```python
from build123d import *

# Parameters (mm, degrees)
SKETCH1_R           = 3.66
BOSS_EXTRUDE1_DEPTH = 1.25
SKETCH2_R           = 2.4
BOSS_EXTRUDE2_DEPTH = 0.8
SKETCH3_R           = 2.25
BOSS_EXTRUDE3_DEPTH = 6.3
BOSS_EXTRUDE4_DEPTH = 2.95
SKETCH5_R           = 0.775
CUT_EXTRUDE4_DEPTH  = 0.2
CUT_EXTRUDE7_DEPTH  = 10.77


with BuildPart() as part:
    # Sketch1 → Boss-Extrude1 (new body)
    with BuildSketch(Plane(origin=(0, 0, 0), x_dir=(1, 0, 0), z_dir=(0, 1, 0))):
        with Locations(Location((0, 0, 0), (0, 0, 270))):
            Circle(SKETCH1_R)
    extrude(amount=BOSS_EXTRUDE1_DEPTH)

    # Sketch2 → Boss-Extrude2 (add)
    with BuildSketch(Plane(origin=(0, 1.25, 0), x_dir=(1, 0, 0), z_dir=(0, 1, 0))):
        with Locations(Location((0, 0, 0), (0, 0, 270))):
            Circle(SKETCH2_R)
    extrude(amount=BOSS_EXTRUDE2_DEPTH)

    # Sketch3 → Boss-Extrude3 (add)
    with BuildSketch(Plane(origin=(0, 2.05, 0), x_dir=(1, 0, 0), z_dir=(0, 1, 0))):
        with Locations(Location((0, 0, 0), (0, 0, 270))):
            Circle(SKETCH3_R)
    extrude(amount=BOSS_EXTRUDE3_DEPTH)

    # Sketch4 → Boss-Extrude4 (add)
    with BuildSketch(Plane(origin=(0, 8.35, 0), x_dir=(1, 0, 0), z_dir=(0, 1, 0))):
        Polygon((-2.222798536, 0), (-1.111399268, -1.925), (1.111399268, -1.925), (2.222798536, 0), (1.111399268, 1.925), (-1.111399268, 1.925), align=None)
    extrude(amount=BOSS_EXTRUDE4_DEPTH)

    # Sketch5 → Cut-Extrude4 (cut)
    with BuildSketch(Plane(origin=(0, 11.3, 0), x_dir=(1, 0, 0), z_dir=(0, 1, 0))):
        with Locations(Location((0, 0, 0), (0, 0, 270))):
            Circle(SKETCH5_R)
    extrude(amount=-CUT_EXTRUDE4_DEPTH, mode=Mode.SUBTRACT)

    # Sketch7 → Cut-Extrude7 (cut)
    with BuildSketch(Plane.XZ):
        Polygon((-0.95, 0), (-0.475, -0.822724134), (0.475, -0.822724134), (0.95, 0), (0.475, 0.822724134), (-0.475, 0.822724134), align=None)
    extrude(amount=-CUT_EXTRUDE7_DEPTH, mode=Mode.SUBTRACT)


solid = part.part
```
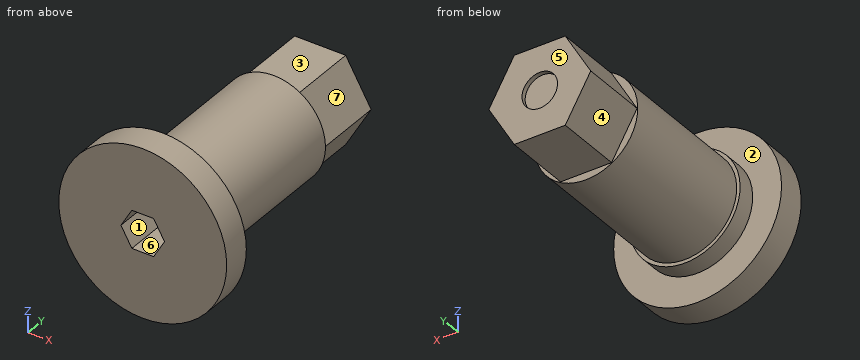
For this review, take the finished solid that the model builds, in its own axes (mm). Face numbers are marked on the shaded views. A direction names the side the tool comes from. Coordinates: 2 decimals unless noted, no trailing zeros. Write each loop counter-clockwise with the first axis right and the second up, starting at its lowest first coordinate (ties: lowest second). Pieces come first, ordered by that corner, then holes. Notation, with made-up numbers: (36, 75) -> (55, 75) arc R17 cw to (55, 94) -> close; hole circle Ø2 at (7.5, -17). An arc over 180 degrees is marked (long way). Put each result on its own line as item: value.
Q1. Take a section at D-D, the plane y = 7.25. State the section outline as (x, z) points (3 decimals), then the cut area to 3 significant figures.
From the geometry:
outline: circle Ø4.5 at (0, 0); hole (-0.95, 0) -> (-0.475, -0.823) -> (0.475, -0.823) -> (0.95, 0) -> (0.475, 0.823) -> (-0.475, 0.823) -> close
area: 13.6 mm2
Q2. Wall thickness on L1, parallel to Y at x = 2.75, z = -0.5; L2, parallel to Y at x = -1.5, z = -1.5; L3, parallel to Z at x = 1.25, y = 5: over which ranges is each line inside the solid? List them lowest first.
From the geometry:
L1: y = 0 to 1.25
L2: y = 0 to 8.35
L3: z = -1.87 to 1.87
Q3. Clearance check with flat-ended pins moving along their axes: pin 1 Ø1.8 at (x, y) = (0.5, 9.5) entering from -Z (3 decimals); pin 2 Ø1 at (x, y) = (0, 4.5) entering from -Z; pin 3 Ø3 at (y, z) = (2.5, 1) entering from -X. State where each tip first meets the part, or that it passes through.
From the geometry:
pin 1: stops at z = -1.925
pin 2: stops at z = -2.25
pin 3: stops at x = -3.66
Q4. Take a section at B-B, the plane x = 0. State the section outline as (y, z) points (3 decimals), then the cut area to 3 significant figures.
From the geometry:
outline: (0, -3.66) -> (1.25, -3.66) -> (1.25, -2.4) -> (2.05, -2.4) -> (2.05, -2.25) -> (8.35, -2.25) -> (8.35, -1.925) -> (11.3, -1.925) -> (11.3, -0.775) -> (11.1, -0.775) -> (11.1, 0.775) -> (11.3, 0.775) -> (11.3, 1.925) -> (8.35, 1.925) -> (8.35, 2.25) -> (2.05, 2.25) -> (2.05, 2.4) -> (1.25, 2.4) -> (1.25, 3.66) -> (0, 3.66) -> (0, 0.823) -> (10.77, 0.823) -> (10.77, -0.823) -> (0, -0.823) -> close
area: 34.7 mm2
Q5. Tool access review of the marked faces 1, 2 and 3: name each direction out of +Z, -Z, +X, -X, +Y, -Y from which nothing blocks a thin tool from reaching the whole face with its end or side.
From the geometry:
face 1: -Y
face 2: +Y
face 3: +Z, +X, -X, +Y
Q6. Take a section at C-C, the plane z = 1.25. State the section outline as (x, y) points.
From the geometry:
outline: (-3.44, 0) -> (3.44, 0) -> (3.44, 1.25) -> (2.05, 1.25) -> (2.05, 2.05) -> (1.87, 2.05) -> (1.87, 8.35) -> (1.5, 8.35) -> (1.5, 11.3) -> (-1.5, 11.3) -> (-1.5, 8.35) -> (-1.87, 8.35) -> (-1.87, 2.05) -> (-2.05, 2.05) -> (-2.05, 1.25) -> (-3.44, 1.25) -> close
Q7. The part is to be moulded in two halves that separate along X. For the marked faces 4, 5, 6 and 7, say which applies: +X half, -X half, draft (parallel to the pull), parting line (faces both ways), or undercut.
From the geometry:
face 4: -X half
face 5: draft
face 6: undercut
face 7: +X half
Q8. Take a section at A-A, the plane y = 10.25. State the section outline as (x, z) points (3 decimals).
From the geometry:
outline: (-2.223, 0) -> (-1.111, -1.925) -> (1.111, -1.925) -> (2.223, 0) -> (1.111, 1.925) -> (-1.111, 1.925) -> close; hole (-0.95, 0) -> (-0.475, -0.823) -> (0.475, -0.823) -> (0.95, 0) -> (0.475, 0.823) -> (-0.475, 0.823) -> close
